Study the drawing (mm; zero at the part's minimum x, y, z) and answer. A direction names the side the tool comes from. Coordinates: 2 decimals unless noted, no trailing zeros. Loops run counter-clockwise (first coordinate to the right, second up) from the corner with the lowest first, then second, coordinate; pieces in that order, holes last.
Q1. Section A-A (z = 30) is taken. Give the vertices of the cut face in (x, y).
Q2. Which of the six approach directions +Z, -Z, +X, -X, +Y, -Y give full straight-line access (tool end or side, diameter ignored) to the marked faces 1 and 2?
Q3. Section C-C (x = 12) is taken. Give the vertices of the cut face in (y, z).
Q4. Section B-B (y = 24.5) is taken. Give the vertices of the cut face in (x, z).
Q5. Flat-ended cylindrical pins translate along their axes: P1, Ø8, axis at y = 40, z = 44.5, coming from the -X side (1 decimal); P2, Ø3.5, axis at y = 59.5, z = 32, coming from the -X side; P3, Ø7.5, axis at y = 31, z = 37.5, coming from the +X side; P4, Ø6, axis at x = 78.5, z = 52.5, coming from the +Y side. Find the tip coordinate at first contact, or state that the pin passes through.
Q6. Straight lines are drawn through the part: line 1 (Z direction, x = 78, y = 53) (1 decimal); line 2 (Y direction, x = 11, z = 34.5) (1 decimal); line 3 (Y direction, x = 36, z = 41.5) (1 decimal). For each, find the intervals that lie inside material, in ascending order.
Q7. Section D-D (x = 69) is taken. Give the vertices of the cut face in (y, z), then the cut area to 3 significant figures.
Q8. The mould has two halves that part along X. Classify the marked faces 3, 4, 5 and 6: pulls with the +X half, pulls with the -X half, needs draft (parallel to the pull), parting line crosses it, or undercut.
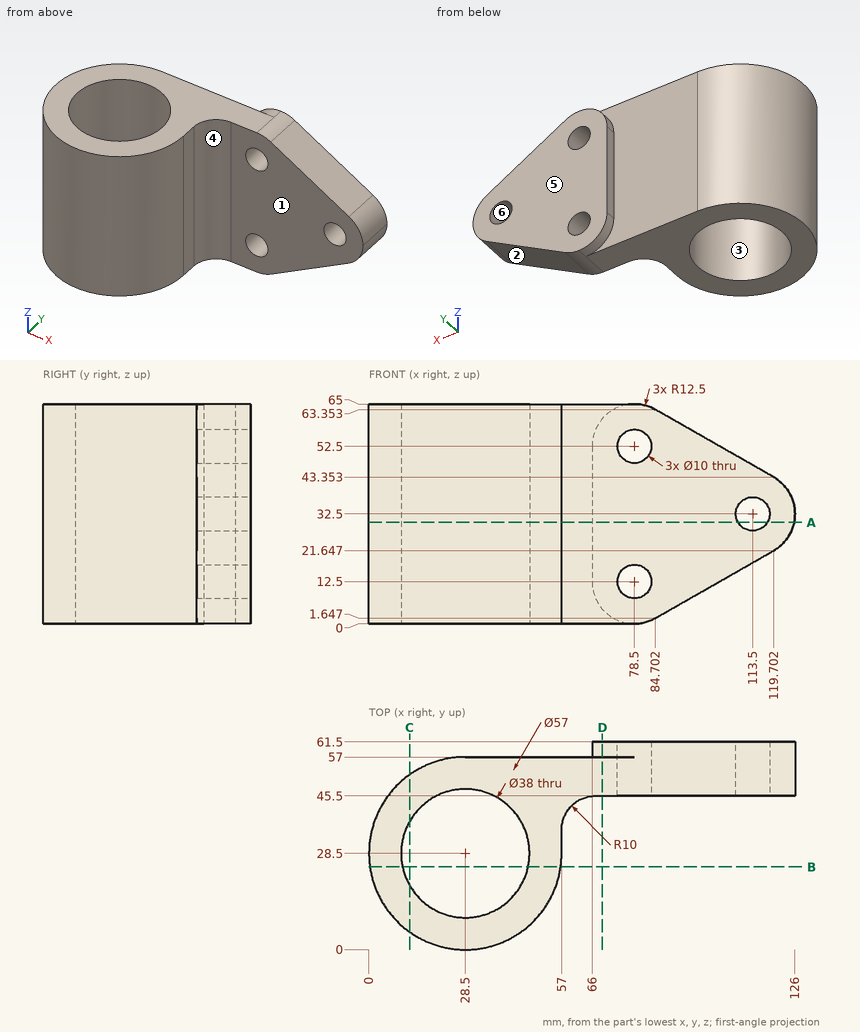
Numbers:
1. outline: (28.5, 57) arc R28.5 ccw (long way) to (57, 28.5) - (57, 35.5) arc R10 cw to (67, 45.5) - (109.17, 45.5) - (109.17, 61.5) - (66, 61.5) - (66, 57) - close; (117.83, 45.5) - (125.75, 45.5) - (125.75, 61.5) - (117.83, 61.5) - close; hole circle Ø38 at (28.5, 28.5)
2. face 1: +Z, -Z, +X, -Y
2. face 2: -Z, +X, +Y, -Y
3. outline: (5.26, 0) - (19.08, 0) - (19.08, 65) - (5.26, 65) - close; (37.92, 0) - (51.74, 0) - (51.74, 65) - (37.92, 65) - close
4. outline: (0.28, 0) - (9.93, 0) - (9.93, 65) - (0.28, 65) - close; (47.07, 0) - (56.72, 0) - (56.72, 65) - (47.07, 65) - close
5. P1: stops at x = 1
5. P2: stops at x = 66
5. P3: stops at x = 57
5. P4: passes through
6. line 1: z = 0 to 7.5, 17.5 to 47.5, 57.5 to 65
6. line 2: y = 6 to 21.1, 35.9 to 51
6. line 3: y = 1 to 11, 46 to 57
7. outline: (45.5, 0) - (57, 0) - (57, 4.38) - (61.5, 4.38) - (61.5, 60.62) - (57, 60.62) - (57, 65) - (45.5, 65) - close
7. area: 1,000 mm2
8. face 3: undercut
8. face 4: pulls with the +X half
8. face 5: needs draft
8. face 6: undercut
